Design review of the part built by this model. Coordinates are the model's own, in mm. Face numbers are marked on the shaded views. A direction names the side the tool comes from. Round coordinates to 2 decimals unless told otherwise and drop trailing zeros. Loops run counter-clockwise (first coordinate to the right, second up) from the corner with the lowest first, then second, coordinate; pieces in that order, holes last. Notation, with made-up numbers: (-35, 30.5) - (-22, 30.5) arc R16 cw to (-22, 59.5) - close; hole circle Ø1 at (-34, 18.25). An arc over 180 degrees is marked (long way). Return JSON: item names as keys, results as strings. Group by question number.
(1) We need section C-C, the plane y = 0.75. Give the number of separate pieces and of enclosed holes in the cut face, and give its area (3 significant figures).
(2) Clearance check with flat-ended pins moving along their axes: pin 1 (0.6 mm diameter, centred on x = 28, y = 1, fed in from +Z); pin 2 (3 mm diameter, centred on x = -29.5, z = 13.5, fed in from +Y); pin 3 (1.8 mm diameter, centred on x = -30.5, z = 0, fed in from -Y); pin 4 (19 mm diameter, centred on x = 24.5, z = -17, fed in from +Y). State where each tip first meets the part, or that it passes through.
(3) We need section D-D, the plane z = -14.5. Write out the cut boundary in (x, y).
(4) For the marked faces 1, 2 and 3, list the 3-axis set-ups (+Z, -Z, +X, -X, +Y, -Y) from which the entire face can be reached by the end or side of a thin tool; tool diameter is ignored.
(5) The part is to be moulded in two halves that separate along X. For the marked faces 4 and 5, say which applies: pulls with the +X half, pulls with the -X half, needs draft (parallel to the pull), parting line crosses it, or undercut.
(6) We need section A-A, the plane x = 0. Write out the cut boundary in (y, z).
(7) Wall thickness on L1, parallel to X at y = 0.6, z = 0; L2, parallel to Z at x = -21, y = 0.9; L3, parallel to Z at x = 22, y = 0.95: over which ranges is each line inside the solid? List them lowest first. Write a range as [from, to].
(8) We need section B-B, the plane z = 0. Write out the cut boundary in (x, y), and give its area (3 significant figures).
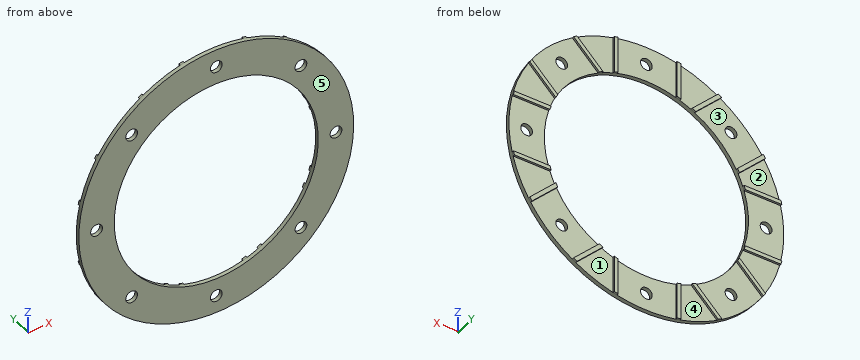
from build123d import *
from build123d.topology import SkipClean

# Parameters (mm, degrees)
SKETCH_1_R               = 35
SKETCH_1_R_2             = 26
SKETCH_1_R_3             = 1.5
EXTRUDE_1_DEPTH          = 1
EXTRUDE_2_DEPTH          = 0.5
PATTERN_CIRCULAR_1_COUNT = 8


with BuildPart() as part:
    # Эскиз1 → Бобышка-Вытянуть1 (new body)
    with BuildSketch(Plane(origin=(0, 0, 0), x_dir=(1, 0, 0), z_dir=(0, 1, 0))):
        with Locations(Location((0, 0, 0), (0, 0, 270))):
            Circle(SKETCH_1_R)
        with Locations(Location((0, 0, 0), (0, 0, 270))):
            Circle(SKETCH_1_R_2, mode=Mode.SUBTRACT)
        with Locations(Location((0, 30.5, 0), (0, 0, 270))):
            Circle(SKETCH_1_R_3, mode=Mode.SUBTRACT)
        with Locations(Location((21.566756826, 21.566756826, 0), (0, 0, 270))):
            Circle(SKETCH_1_R_3, mode=Mode.SUBTRACT)
        with Locations(Location((30.5, 0, 0), (0, 0, 270))):
            Circle(SKETCH_1_R_3, mode=Mode.SUBTRACT)
        with Locations(Location((21.566756826, -21.566756826, 0), (0, 0, 270))):
            Circle(SKETCH_1_R_3, mode=Mode.SUBTRACT)
        with Locations(Location((0, -30.5, 0), (0, 0, 270))):
            Circle(SKETCH_1_R_3, mode=Mode.SUBTRACT)
        with Locations(Location((-21.566756826, -21.566756826, 0), (0, 0, 270))):
            Circle(SKETCH_1_R_3, mode=Mode.SUBTRACT)
        with Locations(Location((-30.5, 0, 0), (0, 0, 270))):
            Circle(SKETCH_1_R_3, mode=Mode.SUBTRACT)
        with Locations(Location((-21.566756826, 21.566756826, 0), (0, 0, 270))):
            Circle(SKETCH_1_R_3, mode=Mode.SUBTRACT)
    extrude(amount=EXTRUDE_1_DEPTH)

    # Эскиз2 → Бобышка-Вытянуть2 (add)
    with SkipClean():  # the faces are left unmerged after this step: merging them gives an invalid solid
        with BuildSketch(Plane(origin=(0, 1, 0), x_dir=(1, 0, 0), z_dir=(0, 1, 0))):
            with BuildLine():
                ThreePointArc((-7.5, 34.186985828), (-8.000861476, 34.0732478), (-8.5, 33.952172243))
                Line((-8.5, 33.952172243), (-8.5, 24.571324751))
                ThreePointArc((-8.5, 24.571324751), (-8.001634558, 24.738105109), (-7.5, 24.894778569))
                Line((-7.5, 24.894778569), (-7.5, 34.186985828))
            make_face()
            with BuildLine():
                ThreePointArc((8.5, 33.952172243), (8.000861476, 34.0732478), (7.5, 34.186985828))
                Line((7.5, 34.186985828), (7.5, 24.894778569))
                ThreePointArc((7.5, 24.894778569), (8.001634558, 24.738105109), (8.5, 24.571324751))
                Line((8.5, 24.571324751), (8.5, 33.952172243))
            make_face()
        extrude_2 = extrude(amount=EXTRUDE_2_DEPTH)

    # Круговой массив1: Бобышка-Вытянуть2 ×8 about axis
    with SkipClean():  # the faces are left unmerged after this step: merging them gives an invalid solid
        pattern_circular_1_axis = Axis((0, 0, 0), (0, 1, 0))
        for i in range(1, PATTERN_CIRCULAR_1_COUNT):
            add(extrude_2.rotate(pattern_circular_1_axis, i * 360 / PATTERN_CIRCULAR_1_COUNT))


solid = part.part
Solutions:
{
 "1": {"separate pieces": "1", "enclosed holes": "9", "area": "1,670 mm^2"},
 "2": {"pin 1": "z = 21.39", "pin 2": "y = 1", "pin 3": "through", "pin 4": "y = 1.5"},
 "3": {"outline": "(-31.86, 0) - (-21.58, 0) - (-21.58, 1) - (-25.11, 1) - (-25.11, 1.5) - (-26.52, 1.5) - (-26.52, 1) - (-31.86, 1) - close; (21.58, 0) - (31.86, 0) - (31.86, 1) - (26.52, 1) - (26.52, 1.5) - (25.11, 1.5) - (25.11, 1) - (21.58, 1) - close"},
 "4": {"face 1": "-Z, +Y", "face 2": "-X, +Y", "face 3": "+Y"},
 "5": {"face 4": "undercut", "face 5": "needs draft"},
 "6": {"outline": "(0, -35) - (1, -35) - (1, -32) - (0, -32) - close; (0, -29) - (1, -29) - (1, -26) - (0, -26) - close; (0, 26) - (1, 26) - (1, 29) - (0, 29) - close; (0, 32) - (1, 32) - (1, 35) - (0, 35) - close"},
 "7": {"L1": "[-35, -32], [-29, -26], [26, 29], [32, 35]", "L2": "[-28, -22.96], [-20.18, -15.33], [15.33, 20.18], [22.96, 28]", "L3": "[-27.22, -23], [-20.13, -13.86], [13.86, 20.13], [23, 27.22]"},
 "8": {"outline": "(-35, 0) - (-32, 0) - (-32, 1) - (-35, 1) - close; (-29, 0) - (-26, 0) - (-26, 1) - (-29, 1) - close; (26, 0) - (29, 0) - (29, 1) - (26, 1) - close; (32, 0) - (35, 0) - (35, 1) - (32, 1) - close", "area": "12.0 mm^2"}
}
